Verification items for the finished model (mm, model axes). Face numbers are marked on the shaded views. A direction names the side the tool comes from. Round coordinates to 2 decimals unless told otherwise and drop trailing zeros. Order: outer loops, then holes, each group sorted by start corner. A loop starts at its lowest first (then second) coordinate and runs counter-clockwise, first axis right, second up. Notation, with made-up numbers: M 39,50 L 67,50 A31 cw 67,81 Z; hole C 78,72 d9. An arc over 180 degrees is marked long. Return JSON: item names as keys, results as strings. Group by question number.
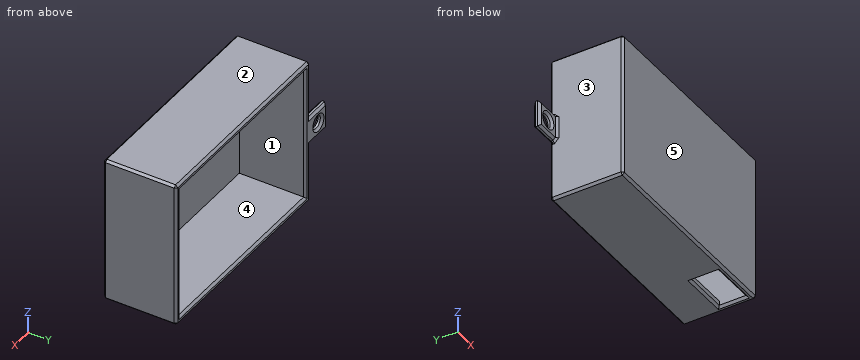
from build123d import *

# Parameters (mm, degrees)
SKETCH_1_W          = 80
SKETCH_1_H          = 50
EXTRUDE_1_DEPTH     = 3
SKETCH_2_W          = 90
SKETCH_2_H          = 60
SKETCH_2_W_2        = 80
SKETCH_2_H_2        = 50
EXTRUDE_3_DEPTH     = 3
SKETCH_2_3_W        = 96
SKETCH_2_3_H        = 66
SKETCH_2_3_W_2      = 90
SKETCH_2_3_H_2      = 60
EXTRUDE_4_DEPTH     = 33
SKETCH_3_W          = 20
SKETCH_3_H          = 12
CUT_EXTRUDE_1_DEPTH = 10
SKETCH_4_R          = 3
EXTRUDE_5_DEPTH     = 3
CHAMFER_1_SIZE      = 1
CHAMFER_2_SIZE      = 1


with BuildPart() as part:
    # 草图1 → 凸台-拉伸1 (new body)
    with BuildSketch(Plane(origin=(0, 0, 0), x_dir=(1, 0, 0), z_dir=(0, 1, 0))):
        with Locations((40, -25)):
            Rectangle(SKETCH_1_W, SKETCH_1_H)
    extrude(amount=EXTRUDE_1_DEPTH)

    # 草图2 → 凸台-拉伸3 (add)
    with BuildSketch(Plane.XZ):
        with Locations((40, 25)):
            Rectangle(SKETCH_2_W, SKETCH_2_H)
        with Locations((40, 25)):
            Rectangle(SKETCH_2_W_2, SKETCH_2_H_2, mode=Mode.SUBTRACT)
    extrude(amount=-EXTRUDE_3_DEPTH)

    # 草图2<3> → 凸台-拉伸4 (add)
    with BuildSketch(Plane.XZ):
        with Locations((40, 25)):
            Rectangle(SKETCH_2_3_W, SKETCH_2_3_H)
        with Locations((40, 25)):
            Rectangle(SKETCH_2_3_W_2, SKETCH_2_3_H_2, mode=Mode.SUBTRACT)
    extrude(amount=-EXTRUDE_4_DEPTH)

    # 草图3 → 切除-拉伸1 (cut)
    with BuildSketch(Plane(origin=(0, 0, -8), x_dir=(-1, 0, 0), z_dir=(0, 0, -1))):
        with Locations((-75, 9)):
            Rectangle(SKETCH_3_W, SKETCH_3_H)
    extrude(amount=-CUT_EXTRUDE_1_DEPTH, mode=Mode.SUBTRACT)

    # 草图4 → 凸台-拉伸5 (add)
    with BuildSketch(Plane(origin=(0, 33, 0), x_dir=(1, 0, 0), z_dir=(0, 1, 0))):
        Polygon((-8, -25), (-8, -19), (-20, -19), (-20, -25), (-20, -31), (-8, -31), align=None)
        with Locations(Location((-14, -25, 0), (0, 0, 270))):
            Circle(SKETCH_4_R, mode=Mode.SUBTRACT)
    extrude(amount=-EXTRUDE_5_DEPTH)

    # 倒角1
    chamfer_1_edges = [part.edges().sort_by_distance(p)[0] for p in [
        (88, 0, 25),
        (40, 0, 58),
        (-8, 0, 25),
        (40, 0, -8),
        (40, 33, 58),
        (-8, 16.5, 58),
        (-8, 33, 44.5),
        (-8, 16.5, -8),
        (40, 33, -8),
        (88, 16.5, -8),
        (88, 33, 25),
        (88, 16.5, 58),
        (85, 33, 25),
        (40, 33, 55),
        (-5, 33, 25),
        (40, 33, -5),
        (85, 9, -8),
        (75, 3, -8),
        (65, 9, -8),
        (75, 15, -8),
        (-8, 33, 5.5),
        (-14, 33, 31),
        (-14, 33, 19),
        (-20, 33, 25),
        (-14, 33, 22),
    ]]
    chamfer(chamfer_1_edges, length=CHAMFER_1_SIZE)

    # 倒角2
    chamfer_2_edges = [part.edges().sort_by_distance(p)[0] for p in [
        (-14, 30, 31),
        (-8, 31, 31),
        (-20, 30, 25),
        (-14, 30, 19),
        (-8, 30, 25),
        (-8, 31, 19),
        (-14, 30, 22),
    ]]
    chamfer(chamfer_2_edges, length=CHAMFER_2_SIZE)


solid = part.part
1. Thickness scan on line 1 along X through (y, z) = (4, 11); line 2 along Z through (x, y) = (47, 24.5); line 3 along Y through (x, z) = (69, 40). Record the ranges inside material, lowest first. Write a range as from..to.
2. Cross-section at A-A (z = 25). Enter the section's corners in (x, y).
3. Cross-section at C-C (y = 18). Enter the section's corners in (x, z), plus the area to 3 significant figures.
4. Cross-section at B-B (x = 70). Enter the section's corners in (y, z), plus the area to 3 significant figures.
5. Go/stop test with flat-tipped pins: pin 1 (5 mm diameter, centred on x = -13.5, z = 23, fed in from -Y); pin 2 (1.1 mm diameter, centred on x = -13.5, y = 31.5, fed in from -Z); pin 3 (0.5 mm diameter, centred on x = -17, y = 31.5, fed in from +Z). Record where each tip stops, or that it passes through.
6. Draft check along X on the marked faces 1, 2 and 3. Enter one of: +X half, -X half, draft (parallel to the pull), parting line (faces both ways), or undercut.
7. Access from +Z, -Z, +X, -X, +Y, -Y to the whole of each face (thin tool, end or side, straight path). Record for the marked faces 4 and 5.
8. Cross-section at D-D (z = 47.5). Enter the section's corners in (x, y), plus the area to 3 significant figures.
Computed:
{
 "1": {"line 1": "x = -8..-5, 85..88", "line 2": "z = -8..-5, 55..58", "line 3": "y = 0..3"},
 "2": {"outline": "M -20,31 L -19,30 L -18,30 L -17,31 L -17,32 L -18,33 L -19,33 L -20,32 Z; M -11,31 L -10,30 L -9,30 L -8,29 L -8,1 L -7,0 L 87,0 L 88,1 L 88,32 L 87,33 L 86,33 L 85,32 L 85,3 L -5,3 L -5,32 L -6,33 L -10,33 L -11,32 Z"},
 "3": {"outline": "M -8,-7 L -7,-8 L 87,-8 L 88,-7 L 88,57 L 87,58 L -7,58 L -8,57 Z; hole M -5,-5 L 85,-5 L 85,55 L -5,55 Z", "area": "934 mm²"},
 "4": {"outline": "M 0,-7 L 1,-8 L 2,-8 L 3,-7 L 3,55 L 32,55 L 33,56 L 33,57 L 32,58 L 1,58 L 0,57 Z; M 15,-7 L 16,-8 L 32,-8 L 33,-7 L 33,-6 L 32,-5 L 15,-5 Z", "area": "338 mm²"},
 "5": {"pin 1": "stops at y = 30", "pin 2": "stops at z = 19", "pin 3": "stops at z = 31"},
 "6": {"face 1": "undercut", "face 2": "draft", "face 3": "-X half"},
 "7": {"face 4": "+Y", "face 5": "+Z, -Z, +X, -X, -Y"},
 "8": {"outline": "M -8,1 L -7,0 L 87,0 L 88,1 L 88,32 L 87,33 L 86,33 L 85,32 L 85,3 L -5,3 L -5,32 L -6,33 L -7,33 L -8,32 Z", "area": "465 mm²"}
}
